Work out the finished part from the listing and answer in its coordinate system (mm). A direction names the side the tool comes from. Coordinates: 2 decimals unless noted, no trailing zeros. Order: outer loops, then holes, each group sorted by start corner. A loop starts at its lowest first (then second) coordinate and runs counter-clockwise, first axis right, second up.
1. Flat-ended cylindrical pins translate along their axes: pin 1 Ø24.5 at (x, y) = (0, 0) entering from -Z; pin 2 Ø3 at (y, z) = (-3.5, 5) entering from -X; pin 3 Ø1.8 at (y, z) = (-13.5, 3) entering from -X; pin 4 Ø3 at (y, z) = (23.5, 3.5) entering from -X. Find the tip coordinate at first contact, or state that the pin passes through.
2. Find the intervals of material crossed by probe 1 along X at (y, z) = (-13, 5.35); probe 2 along Y at (x, z) = (-23, 1.5); probe 3 along Y at (x, z) = (-24, 3.3), in increasing order.
3. Determine the mould class of faces 4 (the flat face through (18.555, -17.963, 2.958)), 5 (the cylindrical face through (10.277, -21.643, 3.042)), 6 (the flat face through (-9, 6, 6)), 7 (the flat face through (-32.407, -11.13, 2.958)) for opening direction Y: +Y half, -Y half, draft (parallel to the pull), parting line (faces both ways), or undercut.
4. The part is cut by section B-B, the plane x = -7.5. Give the vertices of the cut face in (y, z).
5. The part is cut by section A-A, the plane z = 5.1. Count the separate pieces of the cut face and the enclosed holes in it, then the cut area to 3 significant figures.
6. A tool of negligible diameter and unlimited length cuts with its end or side. For faces 1 (the flat face through (-24.75, -17.96, 2.96)), 2 (the flat face through (-26, -22.5, 3)), 3 (the cylindrical face through (-10.207, -21.595, 3.042)), from which of +Z, -Z, +X, -X, +Y, -Y can it reach the whole face along a straight path? Write none if from no direction.
```python
from build123d import *

# Parameters (mm, degrees)
F0_R     = 9.45
F1_DEPTH = 6
F2_R     = 5


with BuildPart() as f1:
    # F0 (on Top) → F1 (new body)
    with BuildSketch(Plane.XY):
        with BuildLine():
            Line((14.9855715851, 19.0442286341), (0, 45))
            Line((0, 45), (-14.9855715851, 19.0442286341))
            ThreePointArc((-14.9855715851, 19.0442286341), (-11.6913429511, 6.75), (-23.9855715851, 3.4557713659))
            Line((-23.9855715851, 3.4557713659), (-38.9711431703, -22.5))
            Line((-38.9711431703, -22.5), (-9, -22.5))
            ThreePointArc((-9, -22.5), (0, -13.5), (9, -22.5))
            Line((9, -22.5), (38.9711431703, -22.5))
            Line((38.9711431703, -22.5), (23.9855715851, 3.4557713659))
            ThreePointArc((23.9855715851, 3.4557713659), (11.6913429511, 6.75), (14.9855715851, 19.0442286341))
        make_face()
        Polygon((-15.3719509172, -16.125), (-21.6506350946, -19.75), (-27.929319272, -16.125), (-27.929319272, -8.875), (-21.6506350946, -5.25), (-15.3719509172, -8.875), align=None, mode=Mode.SUBTRACT)
        Polygon((21.6506350946, -5.25), (27.929319272, -8.875), (27.929319272, -16.125), (21.6506350946, -19.75), (15.3719509172, -16.125), (15.3719509172, -8.875), align=None, mode=Mode.SUBTRACT)
        Circle(F0_R, mode=Mode.SUBTRACT)
        Polygon((-6.2786841774, 28.625), (0, 32.25), (6.2786841774, 28.625), (6.2786841774, 21.375), (0, 17.75), (-6.2786841774, 21.375), align=None, mode=Mode.SUBTRACT)
    extrude(amount=F1_DEPTH)

    # F2
    f2_edges = [f1.edges().sort_by_distance(p)[0] for p in [
        (14.985572, 19.044229, 3),
        (-23.985572, 3.455771, 3),
        (9, -22.5, 3),
        (-14.985572, 19.044229, 3),
        (-9, -22.5, 3),
        (23.985572, 3.455771, 3),
    ]]
    fillet(f2_edges, radius=F2_R)


solid = f1.part
```
Geometry says:
1. pin 1: stops at z = 0
1. pin 2: stops at x = -28.87
1. pin 3: stops at x = -34.29
1. pin 4: stops at x = -13.23
2. probe 1: x = -33.49 to -27.93, -15.37 to 15.37, 27.93 to 33.49
2. probe 2: y = -22.5 to -18.97, -6.03 to 2.25
2. probe 3: y = -22.5 to -18.39, -6.61 to 1.86
3. face 4: undercut
3. face 5: -Y half
3. face 6: draft
3. face 7: +Y half
4. outline: (-17.53, 0) - (-5.75, 0) - (-5.75, 6) - (-17.53, 6) - close; (5.75, 0) - (32.01, 0) - (32.01, 6) - (5.75, 6) - close
5. separate pieces: 1
5. enclosed holes: 4
5. area: 1,540 mm2
6. face 1: +Z, -Z
6. face 2: +Z, -Z, +X, -X, -Y
6. face 3: +Z, -Z, -Y
